CAD build for the part. Positions are in the model's coordinates, mm. Face numbers are marked on the shaded views. A direction names the side the tool comes from. Coordinates: 2 decimals unless noted, no trailing zeros. Write each loop counter-clockwise with the first axis right and the second up, starting at its lowest first coordinate (ties: lowest second). Pieces come first, ordered by that corner, then holes. Notation, with made-up numbers: (80, 71.5) - (136, 71.5) arc R12 ccw to (136, 85.5) - close; hole circle Ø4 at (28, 49.5). An arc over 180 degrees is marked (long way). Answer in a Markdown table with one row per item. Add a question column.
Q1. Band-saw the part on D-D (z = 20). List the corners of the cut face in (x, y) (3 decimals), and give its area (3 significant figures).
Q2. 3-axis set-ups, long thin cutter, end or side, ignore diameter. For the marked faces 1 and 2: which of +Z, -Z, +X, -X, +Y, -Y reach the whole face in a straight line?
Q3. Two-plate mould, pull along Z, no slides. Class the marked faces 3, 4 and 5: +Z half, -Z half, draft (parallel to the pull), parting line (faces both ways), or undercut.
Q4. Drill centre lines: line 1 along Y through (x, z) = (0, 12.25) (3 decimals); line 2 along Y through (x, z) = (0, 12.5). Where is each one in solid material? Low to high. Write a range as from..to.
Q5. Pin check, flat tips, straight feed: pin 1 (1.5 mm diameter, centred on y = 2, z = 12, fed in from +X); pin 2 (1.5 mm diameter, centred on x = 1, z = 2.5, fed in from +Y); pin 3 (1 mm diameter, centred on x = -3.5, y = -6.5, fed in from -Z). Stop position of each tip, or through.
Q6. Band-saw the part on A-A (z = 15.25). List the corners of the cut face in (x, y).
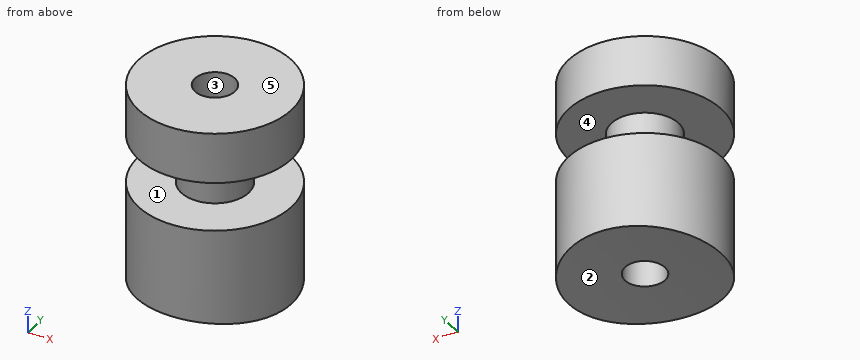
```python
from build123d import *

# Parameters (mm, degrees)
SKETCH1_R              = 9.525
EXTRUDE1_DEPTH         = 24.78278
SKETCH2_OUTSIDE_W      = 28.372
SKETCH2_OUTSIDE_H      = 28.372
SKETCH2_OUTSIDE_R      = 4.191
EXTRUDE2_DEPTH         = 6.096
EXTRUDE3_DEPTH         = 29.207045831
EXTRUDE3_DEPTH_BACK    = 29.207045831
F_10_CLEARANCE_HOLE1_D = 4.9784


with BuildPart() as part:
    # Sketch1 → Extrude1 (new body)
    with BuildSketch(Plane.XY):
        Circle(SKETCH1_R)
    extrude(amount=EXTRUDE1_DEPTH)

    # Sketch2 outside → Extrude2 (cut)
    with BuildSketch(Plane.XY.offset(18.48358)):
        Rectangle(SKETCH2_OUTSIDE_W, SKETCH2_OUTSIDE_H)
        Circle(SKETCH2_OUTSIDE_R, mode=Mode.SUBTRACT)
    extrude(amount=-EXTRUDE2_DEPTH, mode=Mode.SUBTRACT)

    # Sketch3 → Extrude3 (cut, two sides: drawn at the far end of the back side and taken through both)
    with BuildSketch(Plane(origin=(0, 0, 0), x_dir=(1, 0, 0), z_dir=(0, 1, 0)).offset(-EXTRUDE3_DEPTH_BACK)):
        with BuildLine():
            Line((81.364445057, 9.888659405), (9.525, 0))
            ThreePointArc((9.525, 0), (0, -0.652479271), (-9.525, 0))
            Line((-9.525, 0), (-81.364445057, 9.888659405))
            Line((-81.364445057, 9.888659405), (-81.364445057, 154.92233068))
            Line((-81.364445057, 154.92233068), (81.364445057, 154.92233068))
            Line((81.364445057, 154.92233068), (81.364445057, 9.888659405))
        make_face()
    extrude(amount=EXTRUDE3_DEPTH + EXTRUDE3_DEPTH_BACK, mode=Mode.SUBTRACT)

    # #10 Clearance Hole1 (through all)
    with Locations(Plane.XY.offset(24.78278)):
        with Locations((0, 0)):
            Hole(F_10_CLEARANCE_HOLE1_D / 2)


solid = part.part
```
Checked values:
| question | item | result |
|---|---|---|
| 1 | outline | circle Ø19.05 at (0, 0); hole circle Ø4.978 at (0, 0) |
| 1 | area | 266 mm² |
| 2 | face 1 | none |
| 2 | face 2 | -Z, +Y, -Y |
| 3 | face 3 | draft |
| 3 | face 4 | undercut |
| 3 | face 5 | +Z half |
| 4 | line 1 | y = -9.525..-2.489, 2.489..9.525 |
| 4 | line 2 | y = -4.19..-2.49, 2.49..4.19 |
| 5 | pin 1 | stops at x = 9.44 |
| 5 | pin 2 | stops at y = 9.52 |
| 5 | pin 3 | stops at z = 0.54 |
| 6 | outline | circle Ø8.38 at (0, 0); hole circle Ø4.98 at (0, 0) |
